Part model, mm, in its own coordinate system. A direction names the side the tool comes from. Give positions to 0.01 mm unless a question says otherwise; leave off trailing zeros. Write each loop counter-clockwise with the first axis right and the second up, starting at its lowest first coordinate (ties: lowest second). Pieces come first, ordered by that corner, then holes. Notation, with made-up numbers: (14.25, -27) - (60.25, -27) arc R15 ccw to (60.25, -15) - close; hole circle Ø6 at (-21.5, 42.5). An arc over 180 degrees is marked (long way). Answer as a JSON object with one key per item and string values. Group by question number.
Autodesk Inventor part; units mm, degrees
ref_plane "YZ Plane" through (0, 0, 0) normal (1, 0, 0) x (0, 1, 0)
ref_plane "XZ Plane" through (0, 0, 0) normal (0, 1, 0) x (-1, 0, 0)
ref_plane "XY Plane" through (0, 0, 0) normal (0, 0, 1) x (1, 0, 0)
sketch "Sketch1" plane through (0, 0, 0) normal (0, 0, 1) x (1, 0, 0)
  line L0 (-5.45, 1.9) -> (5.45, 1.9)
  line L1 (5.45, 1.9) -> (5.45, -1.9)
  line L2 (5.45, -1.9) -> (-5.45, -1.9)
  line L3 (-5.45, -1.9) -> (-5.45, 1.9)
  point P0 (0, 0)
  dimension "d0" = 10.9
  dimension "d1" = 5.45
  dimension "d2" = 3.8
  dimension "d3" = 1.9
extrude "Extrusion1" add sketch "Sketch1" along normal blind 8.8
chamfer "Chamfer1" distance 2 angle 30 1 edges at (0, -1.9, 0) measured on face at (1.8167, -1.9, 2.9333)
chamfer "Chamfer2" distance 2 angle 30 1 edges at (0, 1.9, 0) measured on face at (-1.8167, 1.9, 2.9333)
sketch "Sketch2" plane through (0, 0, 0) normal (0, 0, -1) x (-1, 0, 0)
  line L0 (5.45, -0.4125) -> (2.65, -0.4125)
  line L1 (2.65, -0.4125) -> (2.65, 0.4125)
  line L2 (2.65, 0.4125) -> (5.45, 0.4125)
  line L3 (5.45, 0.4125) -> (5.45, -0.4125)
  line L4 (5.45, -0.7453) -> (5.45, 0.7453)
  point P0 (0, 0)
  dimension "d12" = 0
  dimension "d13" = 2.8
  dimension "d14" = 0.825
  dimension "d15" = 0.4125
extrude "Extrusion2" add sketch "Sketch2" along normal blind 7.5
chamfer "Chamfer3" distance 4 angle 10 1 edges at (-5.45, 0, -7.5) measured on face at (-5.45, -0.6333, 4.2667)
chamfer "Chamfer4" distance 4 angle 10 1 edges at (-2.65, 0, -7.5) measured on face at (-2.65, -0.1375, -2.5)
chamfer "Chamfer5" distance 2 angle 10 1 edges at (-4.05, -0.4125, -7.5) measured on face at (-3.8184, -0.4125, -4.8333)
chamfer "Chamfer6" distance 2 angle 10 1 edges at (-4.05, 0.4125, -7.5) measured on face at (-3.8184, 0.4125, -4.8333)
sketch "Sketch3" plane through (-5.45, -1.9, 8.8) normal (0, -1, 0) x (1, 0, 0)
  line L0 (0, -6.8) -> (0, 0)
  line L1 (0, -8.8) -> (10.9, -8.8)
  line L2 (0, -0.8922) -> (2.9164, -0.8922)
  line L3 (2.9164, -0.8922) -> (2.9164, -8.8)
  line L4 (2.9164, -8.8) -> (0, -8.8)
  line L5 (0, -8.8) -> (0, -0.8922)
  point P0 (5.45, -8.8)
extrude "Extrusion3" cut sketch "Sketch3" against normal blind 0.5
mirror "Mirror1" about plane through (0, 0, 0) normal (0, 1, 0) of "Extrusion3"
mirror "Mirror2" about plane through (0, 0, 0) normal (1, 0, 0) of "Extrusion3", "Mirror1"
mirror "Mirror3" about plane through (0, 0, 0) normal (1, 0, 0) of "Extrusion2"
chamfer "Chamfer7" distance 4 angle 10 1 edges at (2.65, 0, -7.5) measured on face at (2.65, -0.1375, -2.5)
chamfer "Chamfer8" distance 4 angle 10 1 edges at (5.45, 0, -7.5) measured on face at (5.45, 0.4667, 3.3919)
chamfer "Chamfer9" distance 2 angle 10 1 edges at (4.05, 0.4125, -7.5) measured on face at (3.8184, 0.4125, -4.8333)
chamfer "Chamfer10" distance 2 angle 10 1 edges at (4.05, -0.4125, -7.5) measured on face at (3.8184, -0.4125, -4.8333)
properties part number "Mini-ATC_FUse"
1) Saw through at B-B (x = 1.25). List the corners of the cut face in (y, z), and give its area (3 significant figures).
2) Two-plate mould, pull along X, no slides. Class faces 5 (the flat face through (-5.45, 0, 4)), 6 (the flat face through (2.93, -0.01, -5.08)), 7 (the flat face through (4, 1.4, 5)), 8 (the flat face through (5.17, -0.01, -5.08)): +X half, -X half, draft (parallel to the pull), parting line (faces both ways), or undercut.
3) Saw through at C-C (y = 1.7). List the corners of the cut face in (x, z).
4) Drop flat-ended pins along their axis: P1, Ø1.4, axis at x = 4.5, z = -4, coming from the -Y side; P2, Ø5, axis at x = 3.5, z = -2, coming from the +Y side; P3, Ø0.8, axis at x = -4.5, z = -3, coming from the +Y side. Give the stop position or say it passes through.
5) Saw through at A-A (z = -0.75). List the corners of the cut face in (x, y), and give its area (3 significant figures).
6) Drill centre lines: line 1 along X through (y, z) = (-0.05, -2.75); line 2 along Y through (x, z) = (-3.5, 6); line 3 along X through (y, z) = (-0.25, -4.5). Where is each one in solid material? Low to high. Write a range as from..to.
7) Which spindle directions (+Z, -Z, +X, -X, +Y, -Y) get a long thin tool onto all of the face, cutting with end or side? Do faces 1 (the flat face through (-4, -0.412, -3)), 2 (the flat face through (-2.93, 0.01, -5.08)), 3 (the flat face through (-4, -1.4, 5)), 4 (the flat face through (4, 0.412, -3)). Say none if no direction does.
8) Saw through at D-D (y = -1.2). List the corners of the cut face in (x, z).
Checks:
{
 "1": {"outline": "(-1.9, 2) - (-0.75, 0) - (0.75, 0) - (1.9, 2) - (1.9, 8.8) - (-1.9, 8.8) - close", "area": "31.1 mm2"},
 "2": {"face 5": "-X half", "face 6": "undercut", "face 7": "draft", "face 8": "+X half"},
 "3": {"outline": "(-5.45, 7.91) - (-2.53, 7.91) - (-2.53, 1.65) - (2.53, 1.65) - (2.53, 7.91) - (5.45, 7.91) - (5.45, 8.8) - (-5.45, 8.8) - close"},
 "4": {"P1": "y = -0.41", "P2": "y = 1.03", "P3": "y = 0.41"},
 "5": {"outline": "(-5.45, -0.41) - (-2.65, -0.41) - (-2.65, 0.41) - (-5.45, 0.41) - close; (2.65, -0.41) - (5.45, -0.41) - (5.45, 0.41) - (2.65, 0.41) - close", "area": "4.62 mm2"},
 "6": {"line 1": "-5.45..-2.65, 2.65..5.45", "line 2": "-1.4..1.4", "line 3": "-5.27..-2.83, 2.83..5.27"},
 "7": {"face 1": "-Z, +X, -X, -Y", "face 2": "-Z, +Y, -Y", "face 3": "-Z, -X, -Y", "face 4": "-Z, +X, -X, +Y"},
 "8": {"outline": "(-5.45, 0.79) - (5.45, 0.79) - (5.45, 8.8) - (-5.45, 8.8) - close"}
}
